```python
from build123d import *

# Parameters (mm, degrees)
SKETCH1_W                 = 77.04328
SKETCH1_H                 = 25.4
BOSS_EXTRUDE1_DEPTH       = 6.35
CUT_EXTRUDE1_START        = -2.38125
SKETCH2_W                 = 5.8975
SKETCH2_H                 = 5.8975
CUT_EXTRUDE1_DEPTH        = 2.1764
F_4_CLEARANCE_HOLE1_D     = 3.4544
F_4_CLEARANCE_HOLE1_DEPTH = 6.35
F_4_CLEARANCE_HOLE1_TIP   = 1.037806461
F_4_CLEARANCE_HOLE2_D     = 3.4544
CUT_EXTRUDE2_DEPTH        = 80.109082874
CUT_EXTRUDE3_DEPTH        = 80.109082874
FILLET1_R                 = 1.5875
FILLET2_R                 = 1.478727


with BuildPart() as part:
    # Sketch1 → Boss-Extrude1 (new, symmetric)
    with BuildSketch(Plane.XY):
        with Locations((-38.52164, 0)):
            Rectangle(SKETCH1_W, SKETCH1_H)
    extrude(amount=BOSS_EXTRUDE1_DEPTH, both=True)

    # Sketch2 → Cut-Extrude1 (cut)
    with BuildSketch(Plane(origin=(0, 12.7, 0), x_dir=(1, 0, 0), z_dir=(0, 1, 0)).offset(CUT_EXTRUDE1_START)):
        with Locations((-6.350000199, 1.99e-07)):
            Rectangle(SKETCH2_W, SKETCH2_H)
    extrude(amount=-CUT_EXTRUDE1_DEPTH, mode=Mode.SUBTRACT)

    # #4 Clearance Hole1
    with Locations(Plane(origin=(0, 12.7, 0), x_dir=(1, 0, 0), z_dir=(0, 1, 0))):
        with Locations((-6.350000199, 1.99e-07)):
            Hole(F_4_CLEARANCE_HOLE1_D / 2, depth=F_4_CLEARANCE_HOLE1_DEPTH)
            with Locations((0, 0, -(F_4_CLEARANCE_HOLE1_DEPTH + F_4_CLEARANCE_HOLE1_TIP / 2))):  # 118° drill point
                Cone(0, F_4_CLEARANCE_HOLE1_D / 2, F_4_CLEARANCE_HOLE1_TIP, mode=Mode.SUBTRACT)

    # #4 Clearance Hole2 (through all)
    with Locations(Plane.XY.offset(6.35)):
        with Locations((-62.80658, -6.35), (-71.53783, 0), (-62.80658, 6.35)):
            Hole(F_4_CLEARANCE_HOLE2_D / 2)

    # Sketch8 → Cut-Extrude2 (cut, through all)
    with BuildSketch(Plane(origin=(0, 0, -6.35), x_dir=(-1, 0, 0), z_dir=(0, 0, -1))):
        Polygon((0, 0), (0, -12.7), (57.19953, -12.7), align=None)
    extrude(amount=-CUT_EXTRUDE2_DEPTH, mode=Mode.SUBTRACT)

    # Sketch9 → Cut-Extrude3 (cut, through all)
    with BuildSketch(Plane.XY.offset(6.35)):
        Polygon((-12.7, 3.684857438), (-25.424765, 0.859580456), (-25.424765, 6.35), (-12.7, 6.35), align=None)
        Polygon((-31.774765, -0.550308751), (-50.801588921, -4.774830592), (-50.801588921, 6.35), (-31.774765, 6.35), align=None)
    extrude(amount=-CUT_EXTRUDE3_DEPTH, mode=Mode.SUBTRACT)

    # Fillet1
    fillet1_edges = [part.edges().sort_by_distance(p)[0] for p in [
        (-25.424765, 0.859580456, 0),
        (-25.424765, 6.35, 0),
        (-31.774765, 6.35, 0),
        (-31.774765, -0.550308751, 0),
        (-50.801588921, -4.774830592, 0),
        (-50.801588921, 6.35, 0),
    ]]
    fillet(fillet1_edges, radius=FILLET1_R)

    # Fillet2
    fillet2_edges = [part.edges().sort_by_distance(p)[0] for p in [
        (-12.7, 6.35, 0),
        (-12.7, 3.684857438, 0),
    ]]
    fillet(fillet2_edges, radius=FILLET2_R - 0.0001)  # a hair under: the kernel refuses the full size


solid = part.part
```
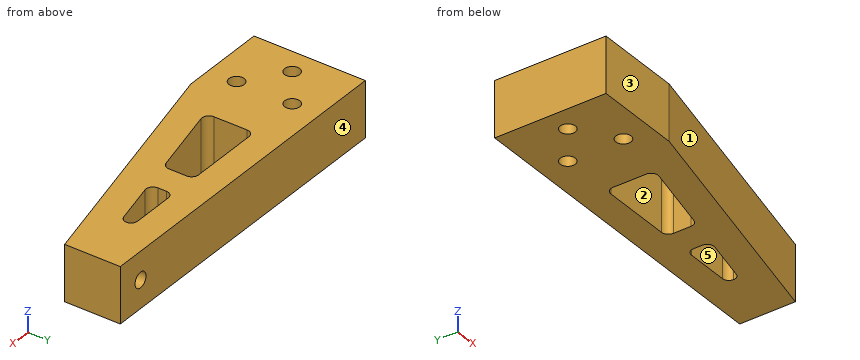
Input: part model. Units: mm. Frame: model coordinates. Face numbers are marked on the shaded views. A direction names the side the tool comes from. Coordinates: 2 decimals unless noted, no trailing zeros. Loops run counter-clockwise (first coordinate to the right, second up) from the corner with the lowest first, then second, coordinate; pieces in that order, holes last.
Q1. Section C-C, the plane y = -6.35. Return the cut outline in (x, z), and give its area (3 significant figures).
Results are:
outline: (-77.04, -6.35) - (-64.53, -6.35) - (-64.53, 6.35) - (-77.04, 6.35) - close; (-61.08, -6.35) - (-28.6, -6.35) - (-28.6, 6.35) - (-61.08, 6.35) - close
area: 571 mm2
Q2. Section B-B, the plane z = 4.75. Give the number of separate pieces and of enclosed holes in the cut face, and give its area (3 significant figures).
Results are:
separate pieces: 1
enclosed holes: 5
area: 1,350 mm2
Q3. Contact query for flat-ended pins moving along their axis: pin 1 (4.5 mm diameter, centred on x = -6, z = 1, fed in from +Y); pin 2 (1.5 mm diameter, centred on x = -36.5, y = 4, fed in from +Z) (1 decimal); pin 3 (2 mm diameter, centred on x = -6.35, z = 0, fed in from +Y); pin 4 (3 mm diameter, centred on x = -6, z = -0.5, fed in from -Y). Output: stop coordinate, or through.
Results are:
pin 1: stops at y = 12.7
pin 2: passes through
pin 3: stops at y = 5.91
pin 4: stops at y = -1.67
Q4. Set-up query: the marked faces 1 and 2. Return all of +Z, -Z, +X, -X, +Y, -Y with unobstructed straight access to the full face (end or side cutting, diameter ignored); none if empty.
Results are:
face 1: +Z, -Z, +X, -Y
face 2: +Z, -Z
Q5. Section A-A, the plane y = 9.25. Return the cut outline in (x, z).
Results are:
outline: (-77.04, -6.35) - (0, -6.35) - (0, 6.35) - (-77.04, 6.35) - close; hole (-9.3, -2.95) - (-3.4, -2.95) - (-3.4, 2.95) - (-9.3, 2.95) - close
Q6. Section D-D, the plane x = -16. Return the cut outline in (y, z).
Results are:
outline: (-3.55, -6.35) - (2.95, -6.35) - (2.95, 6.35) - (-3.55, 6.35) - close; (6.35, -6.35) - (12.7, -6.35) - (12.7, 6.35) - (6.35, 6.35) - close
Q7. Line query: line 1 along X through (y, z) = (4.5, -0.5); line 2 along Y through (x, z) = (-17, -4.25); line 3 along Y through (x, z) = (-25, 0.75). Output: solid intervals per line, ascending.
Results are:
line 1: x = -77.04 to -50.8, -31.77 to -25.42, -12.75 to 0
line 2: y = -3.77 to 2.73, 6.35 to 12.7
line 3: y = -5.55 to 1.76, 5.84 to 12.7
Q8. Mould query, pull axis Y, two halves, no side actions, for the marked faces 3, 4 and 5. Classes: +Y half, -Y half, draft (parallel to the pull), parting line (faces both ways), or undercut.
Results are:
face 3: -Y half
face 4: +Y half
face 5: undercut
